The listing builds one solid part. Answer for the finished solid, in the listing's coordinates (mm). A direction names the side the tool comes from. Give positions to 0.01 mm unless a question says otherwise; leave off trailing zeros. Order: outer loops, then holes, each group sorted by start corner. A loop starts at its lowest first (then second) coordinate and runs counter-clockwise, first axis right, second up.
```python
from build123d import *

# Parameters (mm, degrees)
SKETCH_3_W          = 52.75
SKETCH_3_H          = 44.78
EXTRUDE_1_DEPTH     = 2
HOLE_WIZARD_M2_1_D  = 1.6
CUT_EXTRUDE_START   = 2
SKETCH_3_5_W        = 9.2
SKETCH_3_5_H        = 7.5
SKETCH_3_5_W_2      = 7.5
SKETCH_3_5_H_2      = 9.2
CUT_EXTRUDE_2_DEPTH = 0.5
SKETCH_3_6_W        = 52.75
SKETCH_3_6_H        = 44.78
SKETCH_3_6_W_2      = 49.95
SKETCH_3_6_H_2      = 41.98
EXTRUDE_3_DEPTH     = 8
SKETCH_10_R         = 1
CUT_EXTRUDE_5_DEPTH = 69.574404117
M1_2X0_25_1_D       = 0.95
SKETCH_13_W         = 4.5
SKETCH_13_H         = 9.2
CUT_EXTRUDE_6_DEPTH = 2
SKETCH_14_W         = 9.2
SKETCH_14_H         = 4.5
SKETCH_14_W_2       = 21
CUT_EXTRUDE_7_DEPTH = 2
SKETCH_15_W         = 4.5
SKETCH_15_H         = 7.5
CUT_EXTRUDE_8_DEPTH = 2
M1_2X0_25_2_D       = 0.95


with BuildPart() as part:
    # 草图3 → 凸台-拉伸1 (new body)
    with BuildSketch(Plane.XY):
        with Locations((24.675, 20.69)):
            Rectangle(SKETCH_3_W, SKETCH_3_H)
    extrude(amount=EXTRUDE_1_DEPTH)

    # M2 螺纹孔1 (through all)
    with Locations(Plane(origin=(2.003, 2, 2), x_dir=(1, 0, 0), z_dir=(0, 0, 1))):
        with Locations((0, 0), (45.447, 0), (45.447, 37.357), (0, 37.357), (21.222, 18.3)):
            Hole(HOLE_WIZARD_M2_1_D / 2)

    # 草图3<5> → 切除-拉伸2 (cut)
    with BuildSketch(Plane.XY.offset(CUT_EXTRUDE_START)):
        with Locations((33.523, 37.63)):
            Rectangle(SKETCH_3_5_W, SKETCH_3_5_H)
        with Locations((45.6, 31.7)):
            Rectangle(SKETCH_3_5_W_2, SKETCH_3_5_H_2)
    extrude(amount=-CUT_EXTRUDE_2_DEPTH, mode=Mode.SUBTRACT)

    # 草图3<6> → 凸台-拉伸3 (add)
    with BuildSketch(Plane.XY):
        with Locations((24.675, 20.69)):
            Rectangle(SKETCH_3_6_W, SKETCH_3_6_H)
        with Locations((24.675, 20.69)):
            Rectangle(SKETCH_3_6_W_2, SKETCH_3_6_H_2, mode=Mode.SUBTRACT)
    extrude(amount=EXTRUDE_3_DEPTH)

    # 草图10 → 切除-拉伸5 (cut, through all)
    with BuildSketch(Plane.ZY.offset(1.7)):
        with Locations((3.3, 10.725)):
            Circle(SKETCH_10_R)
    extrude(amount=-CUT_EXTRUDE_5_DEPTH, mode=Mode.SUBTRACT)

    # M1.2x0.25 螺纹孔1 (through all)
    with Locations(Plane.ZY.offset(1.7)):
        with Locations((3.3, 16.775), (3.3, 4.675)):
            Hole(M1_2X0_25_1_D / 2)

    # 草图13 → 切除-拉伸6 (cut)
    with BuildSketch(Plane(origin=(51.05, 0, 0), x_dir=(0, 0, -1), z_dir=(1, 0, 0))):
        with Locations((-4.25, 31.65)):
            Rectangle(SKETCH_13_W, SKETCH_13_H)
    extrude(amount=-CUT_EXTRUDE_6_DEPTH, mode=Mode.SUBTRACT)

    # 草图14 → 切除-拉伸7 (cut)
    with BuildSketch(Plane(origin=(0, 43.08, 0), x_dir=(1, 0, 0), z_dir=(0, 1, 0))):
        with Locations((33.523, -4.25)):
            Rectangle(SKETCH_14_W, SKETCH_14_H)
        with Locations((16.57, -4.25)):
            Rectangle(SKETCH_14_W_2, SKETCH_14_H)
    extrude(amount=-CUT_EXTRUDE_7_DEPTH, mode=Mode.SUBTRACT)

    # 草图15 → 切除-拉伸8 (cut)
    with BuildSketch(Plane.ZY.offset(1.7)):
        with Locations((4.25, 30.2)):
            Rectangle(SKETCH_15_W, SKETCH_15_H)
    extrude(amount=-CUT_EXTRUDE_8_DEPTH, mode=Mode.SUBTRACT)

    # M1.2x0.25 螺纹孔2 (through all)
    with Locations(Plane(origin=(-0.8, -0.8, 8), x_dir=(1, 0, 0), z_dir=(0, 0, 1))):
        with Locations((0, 0), (51.05, 0), (51.05, 43.08), (0, 43.08)):
            Hole(M1_2X0_25_2_D / 2)


solid = part.part
```
1) Given P1, Ø21.5, axis at x = 18.5, y = 23, coming from the +Z side; P2, Ø6, axis at x = 34.5, y = 37.5, coming from the +Z side, each flat-ended and moving along its own axis, determine where each tip first touches the part or whether it passes through.
Geometry says:
P1: stops at z = 2
P2: stops at z = 1.5
2) For a pull along Z with two mould halves and no side action, classify faces 1 (the flat face through (25, 42, 8)), 2 (the cylindrical face through (47.081, 38.647, 0.986)), 3 (the flat face through (28.923, 42, 4)) as +Z half, -Z half, draft (parallel to the pull), parting line (faces both ways), or undercut.
Geometry says:
face 1: +Z half
face 2: draft
face 3: undercut
3) Straight lines are drawn through the part: probe 1 along Y at (x, z) = (47.45, 1.15); probe 2 along X at (y, z) = (42.28, 4) (3 decimals); probe 3 along X at (y, z) = (39, 3.75). For each, find the intervals that lie inside material, in ascending order.
Geometry says:
probe 1: y = -1.7 to 1.2, 2.8 to 38.56, 40.16 to 43.08
probe 2: x = -1.7 to -1.275, -0.325 to 6.07, 27.07 to 28.923, 38.123 to 49.775, 50.725 to 51.05
probe 3: x = -1.7 to -0.3, 49.65 to 51.05
4) Find section D-D (x = 3.5). Write down the section's boundary in (y, z).
Geometry says:
outline: (-1.7, 0) - (43.08, 0) - (43.08, 8) - (41.68, 8) - (41.68, 2) - (-0.3, 2) - (-0.3, 8) - (-1.7, 8) - close
5) Find section A-A (z = 5.5). Write down the section's boundary in (x, y) (3 decimals).
Geometry says:
outline: (-1.7, -1.7) - (51.05, -1.7) - (51.05, 27.05) - (49.65, 27.05) - (49.65, -0.3) - (-0.3, -0.3) - (-0.3, 26.45) - (-1.7, 26.45) - close; (-1.7, 33.95) - (-0.3, 33.95) - (-0.3, 41.68) - (6.07, 41.68) - (6.07, 43.08) - (-1.7, 43.08) - close; (27.07, 41.68) - (28.923, 41.68) - (28.923, 43.08) - (27.07, 43.08) - close; (38.123, 41.68) - (49.65, 41.68) - (49.65, 36.25) - (51.05, 36.25) - (51.05, 43.08) - (38.123, 43.08) - close; hole circle Ø0.95 at (-0.8, -0.8); hole circle Ø0.95 at (-0.8, 42.28); hole circle Ø0.95 at (50.25, -0.8); hole circle Ø0.95 at (50.25, 42.28)
6) Find section C-C (y = 31). Write down the section's boundary in (x, z).
Geometry says:
outline: (-1.7, 0) - (51.05, 0) - (51.05, 2) - (49.35, 2) - (49.35, 1.5) - (41.85, 1.5) - (41.85, 2) - (-1.7, 2) - close; (-1.7, 6.5) - (-0.3, 6.5) - (-0.3, 8) - (-1.7, 8) - close; (49.65, 6.5) - (51.05, 6.5) - (51.05, 8) - (49.65, 8) - close
7) A tool of negligible diameter and unlimited length cuts with its end or side. For faces 4 (the cylindrical face through (22.79, 20.97, 0.99)), 5 (the flat face through (6.07, 42, 4)), 6 (the flat face through (30, 41.68, 7)), 7 (the flat face through (-1, 33.95, 4)), from which of +Z, -Z, +X, -X, +Y, -Y can it reach the whole face along a straight path? Write none if from no direction.
Geometry says:
face 4: +Z, -Z
face 5: +Y
face 6: +Z
face 7: +X, -X
8) Find section B-B (x = 36). Write down the section's boundary in (y, z).
Geometry says:
outline: (-1.7, 0) - (43.08, 0) - (43.08, 2) - (41.38, 2) - (41.38, 1.5) - (33.88, 1.5) - (33.88, 2) - (-0.3, 2) - (-0.3, 8) - (-1.7, 8) - close; (41.68, 6.5) - (43.08, 6.5) - (43.08, 8) - (41.68, 8) - close
